Verification items for the finished model (mm, model axes). A direction names the side the tool comes from. Coordinates: 2 decimals unless noted, no trailing zeros. Write each loop counter-clockwise with the first axis right and the second up, starting at its lowest first coordinate (ties: lowest second). Pieces come first, ordered by that corner, then holes. Notation, with made-up numbers: M 19,-0.5 L 77,-0.5 A26 ccw 77,29.5 Z; hole C -31.75,85 d6. An arc over 180 degrees is marked long. Answer in a Markdown table with one row per item.
from build123d import *

# Parameters (mm, degrees)
BOSS_EXTRUDE1_DEPTH      = 9.525
BOSS_EXTRUDE1_DEPTH_BACK = 9.525
SKETCH2_R                = 12.7
BOSS_EXTRUDE2_DEPTH      = 19.05
SKETCH3_R                = 12.7
BOSS_EXTRUDE3_DEPTH      = 19.05
SKETCH4_R                = 11.1125
CUT_EXTRUDE1_DEPTH       = 19.05
SKETCH5_R                = 11.1125
CUT_EXTRUDE2_DEPTH       = 19.05


with BuildPart() as part:
    # Sketch1 → Boss-Extrude1 (new body, two sides)
    with BuildSketch(Plane.XY) as boss_extrude1_sk:
        Polygon((14.619756732, 5.945361145), (41.514078034, 28.51237623), (-22.164858678, 104.401977829), (-140.313745495, 104.401977829), (-140.313745495, 77.731977829), (-159.363745495, 77.731977829), (-159.363745495, 123.451977829), (-13.281697791, 123.451977829), (68.35232864, 26.164333553), (26.864860696, -8.647785497), align=None)
    extrude(amount=BOSS_EXTRUDE1_DEPTH)
    extrude(boss_extrude1_sk.sketch, amount=-BOSS_EXTRUDE1_DEPTH_BACK)

    # Sketch2 → Boss-Extrude2 (add)
    with BuildSketch(Plane.ZY.offset(159.363745495)):
        with Locations((0, 77.731977829)):
            Circle(SKETCH2_R)
    extrude(amount=-BOSS_EXTRUDE2_DEPTH)

    # Sketch3 → Boss-Extrude3 (add)
    with BuildSketch(Plane(origin=(15.358116398, -18.303090393, 0), x_dir=(0.766044443, 0.64278761, 0), z_dir=(0.64278761, -0.766044443, 0))):
        with Locations((15.020987883, 0)):
            Circle(SKETCH3_R)
    extrude(amount=-BOSS_EXTRUDE3_DEPTH)

    # Sketch4 → Cut-Extrude1 (cut)
    with BuildSketch(Plane(origin=(15.358116398, -18.303090393, 0), x_dir=(0.766044443, 0.64278761, 0), z_dir=(0.64278761, -0.766044443, 0))):
        with Locations((15.020987883, 0)):
            Circle(SKETCH4_R)
    extrude(amount=-CUT_EXTRUDE1_DEPTH, mode=Mode.SUBTRACT)

    # Sketch5 → Cut-Extrude2 (cut)
    with BuildSketch(Plane.ZY.offset(159.363745495)):
        with Locations((0, 77.731977829)):
            Circle(SKETCH5_R)
    extrude(amount=-CUT_EXTRUDE2_DEPTH, mode=Mode.SUBTRACT)


solid = part.part
1) Depth check by flat-ended pin: pin 1 (1.5 mm diameter, centred on x = -6.5, z = 10, fed in from -Y); pin 2 (10 mm diameter, centred on x = 26, y = 89, fed in from -Z); pin 3 (5.5 mm diameter, centred on x = -56, z = 4, fed in from -Y); pin 4 (1.5 mm diameter, centred on y = 33.5, z = 7.5, fed in from +X). Enter the tip coordinate at first touch or a pass-through.
Response values:
| item | result |
|---|---|
| pin 1 | stops at y = 85.04 |
| pin 2 | passes through |
| pin 3 | stops at y = 104.4 |
| pin 4 | stops at x = 62.83 |
2) Thickness scan on L1, parallel to Y at x = -150.25, z = 0; L2, parallel to Y at x = -51.5, z = 8.25; L3, parallel to Z at x = -111, y = 113 (3 decimals). Record the ranges inside material, lowest first. Write a range as [from, to].
Response values:
| item | result |
|---|---|
| L1 | y = [65.03, 66.62], [88.84, 123.45] |
| L2 | y = [104.4, 123.45] |
| L3 | z = [-9.525, 9.525] |
3) Sectioned sample at B-B (z = 3). Record the cut outline in (x, y), then the cut area to 3 significant figures.
Response values:
| item | result |
|---|---|
| outline | M -159.36,65.39 L -140.31,65.39 L -140.31,67.03 L -159.36,67.03 Z; M -159.36,88.43 L -140.31,88.43 L -140.31,104.4 L -22.16,104.4 L 41.51,28.51 L 22.82,12.82 L 35.06,-1.77 L 68.35,26.16 L -13.28,123.45 L -159.36,123.45 Z; M 5.17,-1.99 L 17.41,-16.58 L 18.67,-15.53 L 6.42,-0.93 Z |
| area | 5,860 mm² |
4) Tool access check on faces 4 (the face through (28.948, 5.36, 3.338)), 5 (the face through (-140.314, 89, 0)), 6 (the face through (10.12, 65.926, 0.133)). Record the directions out of +Z, -Z, +X, -X, +Y, -Y that give a thin tool (end or side, any length) a straight path to the whole face; none if there is none.
Response values:
| item | result |
|---|---|
| face 4 | none |
| face 5 | +Z, -Z, -Y |
| face 6 | +Z, -Z |
5) Sectioned sample at D-D (y = 31). Record the cut outline in (x, z) (3 decimals), then the cut area to 3 significant figures.
Response values:
| item | result |
|---|---|
| outline | M 39.427,-9.525 L 64.295,-9.525 L 64.295,9.525 L 39.427,9.525 Z |
| area | 474 mm² |
6) Release check for a two-part mould opening along Y. For faces 1 (the face through (-149.97, 65.04, -0.41)), 2 (the face through (-149.972, 87.102, 5.974)), 3 (the face through (-45, 107, -9.525)) record: +Y half, -Y half, draft (parallel to the pull), parting line (faces both ways), or undercut.
Response values:
| item | result |
|---|---|
| face 1 | parting line |
| face 2 | undercut |
| face 3 | draft |
7) Sectioned sample at C-C (x = -86). Record the cut outline in (y, z) (3 decimals), then the cut area to 3 significant figures.
Response values:
| item | result |
|---|---|
| outline | M 104.402,-9.525 L 123.452,-9.525 L 123.452,9.525 L 104.402,9.525 Z |
| area | 363 mm² |
8) Sectioned sample at A-A (y = 83). Record the cut outline in (x, z) (3 decimals).
Response values:
| item | result |
|---|---|
| outline | M -159.364,-11.556 L -140.314,-11.556 L -140.314,-9.784 L -159.364,-9.784 Z; M -159.364,9.784 L -140.314,9.784 L -140.314,11.556 L -159.364,11.556 Z; M -4.206,-9.525 L 20.662,-9.525 L 20.662,9.525 L -4.206,9.525 Z |
